Could you check a few things on this model? Use its own coordinates, in mm. A direction names the side the tool comes from. Coordinates: 2 decimals unless noted, no trailing zeros. Loops run counter-clockwise (first coordinate to the right, second up) from the corner with the lowest first, then second, coordinate; pieces in that order, holes last.
Autodesk Fusion 360 part; units mm, degrees
sketch "Sketch1" plane through (0, 0, 0) normal (0, 0, 1) x (1, 0, 0)
  line L0 (0, 0) -> (20, 0)
  line L1 (20, 0) -> (120, -250)
  line L2 (120, -250) -> (70, -400)
  line L3 (70, -400) -> (50, -400)
  line L4 (4, -10) -> (14, -10)
  line L5 (53.3333, -390) -> (63.3333, -390)
  line L6 (63.3333, -386) -> (54.6667, -386)
  line L7 (100, -250) -> (54.6667, -386)
  line L8 (53.3333, -390) -> (50, -400)
  line L9 (0, 0) -> (4, -10)
  line L10 (5.6, -14) -> (100, -250)
  line L11 (14, -10) -> (14, -14)
  line L12 (5.6, -14) -> (14, -14)
  line L13 (63.3333, -390) -> (63.3333, -386)
  dimension "d4" = 400
  dimension "d5" = 50
  dimension "d6" = 50
  dimension "d7" = 250
  dimension "d9" = 20
  dimension "d10" = 20
  dimension "d11" = 20
  dimension "d12" = 10
  dimension "d13" = 4
  dimension "d14" = 10
  dimension "d15" = 10
  dimension "d16" = 4
  dimension "d17" = 10
  dimension "d27" = 4
extrude "Extrude1" add sketch "Sketch1" along normal blind 4
sketch "Sketch1 (2)" plane through (0, 0, 0) normal (0, 0, 1) x (1, 0, 0) in component "Lampi1"
component "Lampi1" placed x (1, 0, 0) y (0, 1, 0) z (0, 0, 1) at (0, 0, 0)
equation "d4 = haed_skerms"
equation "d5 = umfram_radius"
equation "d6 = umfram_radius"
equation "d7 = haed_u"
equation "d9 = Linear Dimension-6"
equation "d10 = Linear Dimension-7"
equation "d11 = Linear Dimension-8"
equation "d12 = dypt_pressfit"
equation "d13 = Linear Dimension-10"
equation "d14 = dypt_pressfit"
equation "d15 = dypt_pressfit"
equation "d16 = Linear Dimension-13"
equation "d17 = dypt_pressfit"
equation "haed_skerms = 400 mm"
equation "haed_u = 250 mm"
equation "head_l = 150 mm"
equation "dypt_pressfit = 10 mm"
equation "umfram_radius = 50 mm"

Autodesk Fusion 360 part; units mm, degrees
sketch "Sketch1" plane through (0, 0, 0) normal (0, 0, 1) x (1, 0, 0)
  circle A0 centre (0, 0) radius 25
  line L0 (49.96, 2) -> (39.96, 2)
  line L1 (39.96, 2) -> (39.96, -2)
  line L2 (39.96, -2) -> (49.96, -2)
  line L3 (44.1446, 23.4788) -> (35.1349, 19.1399)
  line L4 (36.8705, 15.536) -> (45.8802, 19.8749)
  line L5 (35.1349, 19.1399) -> (36.8705, 15.536)
  line L6 (29.5859, 40.3073) -> (23.351, 32.489)
  line L7 (26.4783, 29.995) -> (32.7132, 37.8133)
  line L8 (23.351, 32.489) -> (26.4783, 29.995)
  line L9 (9.1673, 49.1524) -> (6.9421, 39.4031)
  line L10 (10.8418, 38.5131) -> (13.067, 48.2623)
  line L11 (6.9421, 39.4031) -> (10.8418, 38.5131)
  line L12 (-13.067, 48.2623) -> (-10.8418, 38.5131)
  line L13 (-6.9421, 39.4031) -> (-9.1673, 49.1524)
  line L14 (-10.8418, 38.5131) -> (-6.9421, 39.4031)
  line L15 (-32.7132, 37.8133) -> (-26.4783, 29.995)
  line L16 (-23.351, 32.489) -> (-29.5859, 40.3073)
  line L17 (-26.4783, 29.995) -> (-23.351, 32.489)
  line L18 (-45.8802, 19.8749) -> (-36.8705, 15.536)
  line L19 (-35.1349, 19.1399) -> (-44.1446, 23.4788)
  line L20 (-36.8705, 15.536) -> (-35.1349, 19.1399)
  line L21 (-49.96, -2) -> (-39.96, -2)
  line L22 (-39.96, 2) -> (-49.96, 2)
  line L23 (-39.96, -2) -> (-39.96, 2)
  line L24 (-44.1446, -23.4788) -> (-35.1349, -19.1399)
  line L25 (-36.8705, -15.536) -> (-45.8802, -19.8749)
  line L26 (-35.1349, -19.1399) -> (-36.8705, -15.536)
  line L27 (-29.5859, -40.3073) -> (-23.351, -32.489)
  line L28 (-26.4783, -29.995) -> (-32.7132, -37.8133)
  line L29 (-23.351, -32.489) -> (-26.4783, -29.995)
  line L30 (-9.1673, -49.1524) -> (-6.9421, -39.4031)
  line L31 (-10.8418, -38.5131) -> (-13.067, -48.2623)
  line L32 (-6.9421, -39.4031) -> (-10.8418, -38.5131)
  line L33 (13.067, -48.2623) -> (10.8418, -38.5131)
  line L34 (6.9421, -39.4031) -> (9.1673, -49.1524)
  line L35 (10.8418, -38.5131) -> (6.9421, -39.4031)
  line L36 (32.7132, -37.8133) -> (26.4783, -29.995)
  line L37 (23.351, -32.489) -> (29.5859, -40.3073)
  line L38 (26.4783, -29.995) -> (23.351, -32.489)
  line L39 (45.8802, -19.8749) -> (36.8705, -15.536)
  line L40 (35.1349, -19.1399) -> (44.1446, -23.4788)
  line L41 (36.8705, -15.536) -> (35.1349, -19.1399)
  arc A1 (49.96, 2) -> (45.8802, 19.8749) centre (0, 0) ccw
  arc A2 (44.1446, 23.4788) -> (32.7132, 37.8133) centre (0, 0) ccw
  arc A3 (29.5859, 40.3073) -> (13.067, 48.2623) centre (0, 0) ccw
  arc A4 (9.1673, 49.1524) -> (-9.1673, 49.1524) centre (0, 0) ccw
  arc A5 (-13.067, 48.2623) -> (-29.5859, 40.3073) centre (0, 0) ccw
  arc A6 (-32.7132, 37.8133) -> (-44.1446, 23.4788) centre (0, 0) ccw
  arc A7 (-45.8802, 19.8749) -> (-49.96, 2) centre (0, 0) ccw
  arc A8 (-49.96, -2) -> (-45.8802, -19.8749) centre (0, 0) ccw
  arc A9 (-44.1446, -23.4788) -> (-32.7132, -37.8133) centre (0, 0) ccw
  arc A10 (-29.5859, -40.3073) -> (-13.067, -48.2623) centre (0, 0) ccw
  arc A11 (-9.1673, -49.1524) -> (9.1673, -49.1524) centre (0, 0) ccw
  arc A12 (13.067, -48.2623) -> (29.5859, -40.3073) centre (0, 0) ccw
  arc A13 (32.7132, -37.8133) -> (44.1446, -23.4788) centre (0, 0) ccw
  arc A14 (45.8802, -19.8749) -> (49.96, -2) centre (0, 0) ccw
  dimension "d1" = 100
  dimension "d6" = 50
  dimension "d7" = 10
  dimension "d8" = 10
  dimension "d9" = 4
  dimension "d11" = 360
extrude "Extrude1" add sketch "Sketch1" along normal blind 4
equation "d1 = D_o"
equation "D_o = 100 mm"
equation "D_i = 50 mm"
equation "offset = 10 mm"
equation "d6 = D_i"
equation "d7 = offset"
equation "d8 = offset"
equation "d9 = Linear Dimension-4"
(1) We'd pull the mould along X, two halves only. Please class faces 1 (the face through (21.81, -44.992, 1.972)), 2 (the face through (26.51, 36.45, 1.97)), 3 (the face through (0, -50, 2)): +X half, -X half, draft (parallel to the pull), parting line (faces both ways), or undercut.
Answers:
face 1: +X half
face 2: undercut
face 3: parting line
(2) I need wall thicknesses on probe 1 along Y at (x, z) = (0, 1.75); probe 2 along X at (y, z) = (42.5, 1.05); probe 3 along X at (y, z) = (-6.5, 2.4). Which ranges of each line are inside material? Lowest first, please.
Answers:
probe 1: y = -50 to -25, 25 to 50
probe 2: x = -26.34 to -11.75, -7.65 to 7.65, 11.75 to 26.34
probe 3: x = -49.58 to -24.14, 24.14 to 49.58
(3) Imagine slicing it at A-A, the plane x = 0. Write out the boundary of the cut face in (y, z).
Answers:
outline: (-50, 0) - (-25, 0) - (-25, 4) - (-50, 4) - close; (25, 0) - (50, 0) - (50, 4) - (25, 4) - close
(4) Imagine slicing it at D-D, the plane y = 35. Write out the boundary of the cut face in (x, z).
Answers:
outline: (-35.71, 0) - (-30.47, 0) - (-30.47, 4) - (-35.71, 4) - close; (-25.35, 0) - (25.35, 0) - (25.35, 4) - (-25.35, 4) - close; (30.47, 0) - (35.71, 0) - (35.71, 4) - (30.47, 4) - close
(5) For pin 1 (1.2 mm diameter, centred on x = 44.5, z = 1.5, fed in from -Y); pin 2 (2 mm diameter, centred on x = -43, z = 2.5, fed in from +Y); pin 3 (1.2 mm diameter, centred on y = -0.5, z = 1.5, fed in from -X); pin 4 (1 mm diameter, centred on x = 28.5, y = -11.5, fed in from -Z), each with a flat end and sliding along its axis, tell me the tip position at first contact or that it passes through.
Answers:
pin 1: stops at y = -23.93
pin 2: stops at y = 27.13
pin 3: stops at x = -39.96
pin 4: stops at z = 0
(6) Imagine slicing it at C-C, the plane x = 42. Write out the boundary of the cut face in (y, z).
Answers:
outline: (-27.13, 0) - (-22.45, 0) - (-22.45, 4) - (-27.13, 4) - close; (-18.01, 0) - (-2, 0) - (-2, 4) - (-18.01, 4) - close; (2, 0) - (18.01, 0) - (18.01, 4) - (2, 4) - close; (22.45, 0) - (27.13, 0) - (27.13, 4) - (22.45, 4) - close
(7) Imagine slicing it at B-B, the plane y = 0. Write out the boundary of the cut face in (x, z).
Answers:
outline: (-39.96, 0) - (-25, 0) - (-25, 4) - (-39.96, 4) - close; (25, 0) - (39.96, 0) - (39.96, 4) - (25, 4) - close
(8) Which directions (+Z, -Z, +X, -X, +Y, -Y) give clear straight access to the entire face, cutting with the end or side of a thin tool? Please do faces 4 (the face through (-39.172, 31.073, 1.972)), 5 (the face through (8.07, 44.35, 1.97)), 6 (the face through (11.94, 43.32, 1.97)).
Answers:
face 4: +Z, -Z, -X, +Y
face 5: +Z, -Z
face 6: +Z, -Z, +Y
